Autodesk Inventor part; units mm, degrees
ref_plane "YZ Plane" through (0, 0, 0) normal (1, 0, 0) x (0, 1, 0)
ref_plane "XZ Plane" through (0, 0, 0) normal (0, 1, 0) x (-1, 0, 0)
ref_plane "XY Plane" through (0, 0, 0) normal (0, 0, 1) x (1, 0, 0)
sketch "Skizze1" plane through (0, 0, 0) normal (0, 1, 0) x (-1, 0, 0)
  circle A0 centre (0, 4) radius 2.1
  circle A1 centre (0, -4) radius 2.1
  line L0 (0, 4) -> (0, -4) construction
  line L1 (0, 4) -> (0, -4) construction
  line L2 (-5.1, 4) -> (-5.1, -4)
  line L3 (5.1, -4) -> (5.1, 4)
  arc A2 (5.1, 4) -> (-5.1, 4) centre (0, 4) ccw
  arc A3 (-5.1, -4) -> (5.1, -4) centre (0, -4) ccw
  point P0 (0, 0)
  point P1 (0, 0)
  point P2 (0, 0)
  dimension "d0" = 4.2
  dimension "d1" = 3
  dimension "d2" = 8
extrude "Extrusion1" add sketch "Skizze1" along normal blind 3
sketch "Skizze2" plane through (0, 0, 0) normal (0, -1, 0) x (1, 0, 0)
  arc A0 (5.1, 4) -> (-5.1, 4) centre (0, 4) ccw construction
  line L0 (3.7094, 7.5) -> (-3.7094, 7.5)
  arc A1 (3.7094, 7.5) -> (-3.7094, 7.5) centre (0, 4) ccw
  arc A2 (5.1, 4) -> (-5.1, 4) centre (0, 4) ccw
  point P0 (0, 0)
  dimension "d5" = 3.5
extrude "Extrusion2" cut sketch "Skizze2" against normal blind 10
properties part number "_3D-Druck"
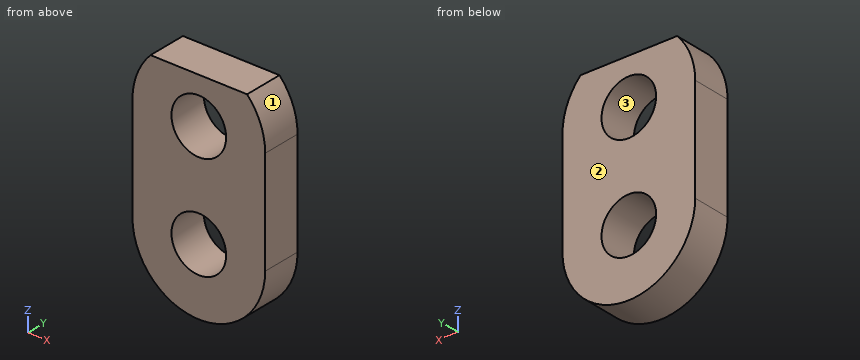
Geometry: final body of the model. Coordinates: model frame, mm. Face numbers are marked on the shaded views. Give positions to 0.01 mm unless a question says otherwise; leave off trailing zeros. Loops run counter-clockwise (first coordinate to the right, second up) from the corner with the lowest first, then second, coordinate; pieces in that order, holes last. Notation, with made-up numbers: (70.25, -1.5) - (116.25, -1.5) arc R26 ccw to (116.25, 19.5) - close; hole circle Ø9 at (-30, 0.5). An arc over 180 degrees is marked (long way). One line per question, with ' | ' between items. Start each with the question number.
(1) Ray query, line 1 (Z direction, x = 0, y = 1.8); line 2 (Z direction, x = -1, y = 0.95); line 3 (X direction, y = 1.45, z = -2.5). Return the intervals inside material, ascending. Write a range as from..to.
(2) Section query B-B on z = 3. Return loops of the section in (x, y), then the cut area to 3 significant figures.
(3) Section query C-C on y = 1.65. Return loops of the section in (x, z).
(4) Section query D-D on z = 5.75. Return loops of the section in (x, y).
(5) Section query A-A on x = 0. Return loops of the section in (y, z), then the cut area to 3 significant figures.
(6) Pull-direction query (Z, two-part tool) for the marked faces 1, 2 and 3; classes: released by +Z, released by -Z, zero draft, split by the parting line, or undercut.
The answers:
1) line 1: -9.1..-6.1, -1.9..1.9, 6.1..7.5 | line 2: -9..-5.85, -2.15..2.15, 5.85..7.5 | line 3: -5.1..-1.47, 1.47..5.1
2) outline: (-5.1, 0) - (-1.85, 0) - (-1.85, 3) - (-5.1, 3) - close; (1.85, 0) - (5.1, 0) - (5.1, 3) - (1.85, 3) - close | area: 19.5 mm2
3) outline: (-5.1, -4) arc R5.1 ccw to (5.1, -4) - (5.1, 4) arc R5.1 ccw to (3.71, 7.5) - (-3.71, 7.5) arc R5.1 ccw to (-5.1, 4) - close; hole circle Ø4.2 at (0, -4); hole circle Ø4.2 at (0, 4)
4) outline: (-4.79, 0) - (-1.16, 0) - (-1.16, 3) - (-4.79, 3) - close; (1.16, 0) - (4.79, 0) - (4.79, 3) - (1.16, 3) - close
5) outline: (0, -9.1) - (3, -9.1) - (3, -6.1) - (0, -6.1) - close; (0, -1.9) - (3, -1.9) - (3, 1.9) - (0, 1.9) - close; (0, 6.1) - (3, 6.1) - (3, 7.5) - (0, 7.5) - close | area: 24.6 mm2
6) face 1: released by +Z | face 2: zero draft | face 3: undercut
